Verification items for the finished model (mm, model axes). Face numbers are marked on the shaded views. A direction names the side the tool comes from. Coordinates: 2 decimals unless noted, no trailing zeros. Loops run counter-clockwise (first coordinate to the right, second up) from the corner with the lowest first, then second, coordinate; pieces in that order, holes last. Notation, with made-up numbers: (5.25, 9) -> (64.25, 9) arc R24 ccw to (64.25, 46) -> close; hole circle Ø4 at (-2.5, 35). An arc over 180 degrees is marked (long way). Use CSV: the item, a comma, the result in double quotes. Start each with the question number.
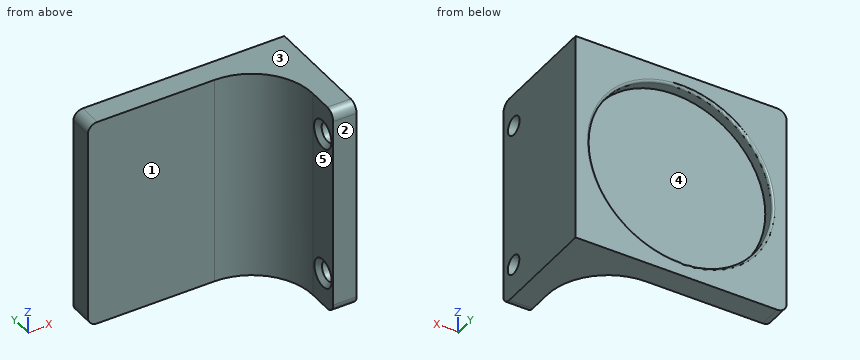
Autodesk Fusion 360 part; units mm, degrees
sketch "Schizzo1" plane through (0, 0, 0) normal (0, 0, 1) x (1, 0, 0)
  line L0 (-8, 11.6314) -> (37, 11.6314)
  line L1 (37, 11.6314) -> (37, -13.3686)
  line L2 (37, -13.3686) -> (32, -13.3686)
  line L3 (32, -13.3686) -> (32, -6.3686)
  line L4 (-8, 11.6314) -> (-8, 6.6314)
  line L5 (-8, 6.6314) -> (19, 6.6314)
  arc A0 (32, -6.3686) -> (19, 6.6314) centre (19, -6.3686) ccw
  dimension "d1" = 5
  dimension "d2" = 5
  dimension "d3" = 45
  dimension "d4" = 25
  dimension "d5" = 13
extrude "Estrusione1" add sketch "Schizzo1" along normal blind 45
fillet "Raccordo1" radius 2 4 edges at (-8, 9.1314, 0) (-8, 9.1314, 45) (34.5, -13.3686, 45) (34.5, -13.3686, 0)
sketch "Schizzo2" plane through (32, 0, 0) normal (-1, 0, 0) x (0, -1, 0)
  arc A0 (11.3686, 0) -> (13.3686, 2) centre (11.3686, 2) ccw
  line L0 (13.3686, 2) -> (13.3686, 43)
  arc A1 (13.3686, 43) -> (11.3686, 45) centre (11.3686, 43) ccw
  line L1 (11.3686, 45) -> (6.3686, 45)
  line L2 (6.3686, 45) -> (6.3686, 0)
  line L3 (6.3686, 0) -> (11.3686, 0)
  line L4 (9.8686, 7.0001) -> (6.3686, 7.0001) construction
  line L5 (9.8686, 7.0001) -> (13.3686, 7.0001) construction
  line L6 (9.7764, 37.9999) -> (6.3686, 37.9999) construction
  line L7 (9.7764, 37.9999) -> (13.1842, 37.9999) construction
  line L8 (9.7764, 37.9999) -> (9.7764, 45) construction
  line L9 (9.8686, 7.0001) -> (9.8686, 0) construction
  point P0 (9.8686, 7.0001)
  point P1 (9.7764, 37.9999)
hole "Foratura1" at (32, -9.8686, 7.0001) at (32, -9.7764, 37.9999) direction (1, 0, 0) diameter 4 depth 11 tip angle 118 countersink diameter 6 countersink angle 90
sketch "Schizzo4" plane through (0, 11.6314, 0) normal (0, 1, 0) x (-1, 0, 0)
  arc A0 (8, 43) -> (6, 45) centre (6, 43) ccw
  line L0 (6, 45) -> (-37, 45)
  line L1 (-37, 45) -> (-37, 0)
  line L2 (-37, 0) -> (6, 0)
  arc A1 (6, 0) -> (8, 2) centre (6, 2) ccw
  line L3 (8, 2) -> (8, 43)
  circle A2 centre (-14.5, 22.5) radius 19.5
  dimension "d19" = 39
  dimension "d20" = 22.5
  dimension "d21" = 22.5
  dimension "d22" = 22.5
  dimension "d23" = 22.5
extrude "Estrusione2" cut sketch "Schizzo4" against normal blind 2.5 contours A2
fillet "Raccordo2" radius 0.5 1 edges at (32.6804, 11.6314, 29.5515)
1. Release check for a two-part mould opening along Z. For the marked faces 3, 4 and 5 record: released by +Z, released by -Z, zero draft, split by the parting line, or undercut.
2. Cross-section at A-A, the plane z = 22.5. Record the boundary of the cut face in (x, y).
3. Set-up check for the marked faces 1 and 2: record each of +Z, -Z, +X, -X, +Y, -Y from which the full face is reachable in a straight line by a thin tool's end or side.
4. Depth check by flat-ended pin: pin 1 (2 mm diameter, centred on y = -9.5, z = 13.5, fed in from -X); pin 2 (19.5 mm diameter, centred on x = 10, z = 18, fed in from +Y). Enter the tip coordinate at first touch or a pass-through.
5. Scan lines: line 1 (Z direction, x = 14.5, y = 9.6); line 2 (Y direction, x = 17.5, z = 32); line 3 (X direction, y = -6.5, z = 24). Record each from-to range of solid material in increasing order.
6. Cross-section at B-B, the plane x = 14.5. Record the boundary of the cut face in (y, z).
Solution:
1,face 3,"released by +Z"
1,face 4,"undercut"
1,face 5,"zero draft"
2,outline,"(-8, 6.63) -> (19, 6.63) arc R13 cw to (32, -6.37) -> (32, -13.37) -> (37, -13.37) -> (37, 11.63) -> (34.5, 11.63) arc R0.5 ccw to (34, 11.13) -> (34, 9.13) -> (-5, 9.13) -> (-5, 11.13) arc R0.5 ccw to (-5.5, 11.63) -> (-8, 11.63) -> close"
3,face 1,"+Z, -Z, -X, -Y"
3,face 2,"+Z, -Z, +X, -X, -Y"
4,pin 1,"stops at x = 32"
4,pin 2,"stops at y = 9.13"
5,line 1,"z = 0 to 3, 42 to 45"
5,line 2,"y = 6.63 to 9.13"
5,line 3,"x = 32 to 37"
6,outline,"(6.63, 0) -> (11.63, 0) -> (11.63, 2.5) arc R0.5 ccw to (11.13, 3) -> (9.13, 3) -> (9.13, 42) -> (11.13, 42) arc R0.5 ccw to (11.63, 42.5) -> (11.63, 45) -> (6.63, 45) -> close"
